Autodesk Inventor part; units mm, degrees
ref_plane "YZ Plane" through (0, 0, 0) normal (1, 0, 0) x (0, 1, 0)
ref_plane "XZ Plane" through (0, 0, 0) normal (0, 1, 0) x (-1, 0, 0)
ref_plane "XY Plane" through (0, 0, 0) normal (0, 0, 1) x (1, 0, 0)
sketch "Sketch1" plane through (0, 0, 0) normal (1, 0, 0) x (0, 1, 0)
  arc A0 (3.7081, 1.5) -> (3.7081, -1.5) centre (0, 0) ccw
  arc A1 (6.5427, 1.6009) -> (8.0964, 0.4688) centre (7.99, 1.955) ccw
  arc A2 (8.0964, -0.4688) -> (6.5427, -1.6009) centre (7.99, -1.955) ccw
  arc A3 (8.0964, -0.4688) -> (8.0964, 0.4688) centre (8.13, 0) ccw
  arc A4 (5.0493, 4.458) -> (6.9512, 4.1777) centre (6.1663, 5.4442) ccw
  arc A5 (7.3869, 3.3475) -> (6.9512, 4.1777) centre (7.1988, 3.7782) ccw
  arc A6 (7.3869, 3.3475) -> (6.5372, 1.623) centre (7.9833, 1.9821) ccw
  arc A7 (2.3992, 6.2939) -> (4.2135, 6.9295) centre (2.9299, 7.6862) ccw
  arc A8 (4.9851, 6.3969) -> (4.2135, 6.9295) centre (4.6184, 6.6909) ccw
  arc A9 (4.9851, 6.3969) -> (5.0342, 4.4751) centre (6.1478, 5.4651) ccw
  arc A10 (-0.8006, 6.688) -> (0.5105, 8.0939) centre (-0.9777, 8.1674) ccw
  arc A11 (1.4413, 7.9809) -> (0.5105, 8.0939) centre (0.98, 8.0707) ccw
  arc A12 (1.4413, 7.9809) -> (2.3778, 6.302) centre (2.9038, 7.6961) ccw
  arc A13 (-3.8169, 5.5498) -> (-3.3094, 7.4041) centre (-4.6612, 6.7775) ccw
  arc A14 (-2.4327, 7.7365) -> (-3.3094, 7.4041) centre (-2.8829, 7.6017) ccw
  arc A15 (-2.4327, 7.7365) -> (-0.8232, 6.6852) centre (-1.0053, 8.164) ccw
  arc A16 (-5.9589, 3.1403) -> (-6.3711, 5.018) centre (-7.277, 3.835) ccw
  arc A17 (-5.7494, 5.7198) -> (-6.3711, 5.018) centre (-6.0854, 5.3912) ccw
  arc A18 (-5.7494, 5.7198) -> (-3.8357, 5.5369) centre (-4.6842, 6.7617) ccw
  arc A19 (-6.7357, 0.0114) -> (-7.9734, 1.4824) centre (-8.2257, 0.0139) ccw
  arc A20 (-7.749, 2.3928) -> (-7.9734, 1.4824) centre (-7.8938, 1.9456) ccw
  arc A21 (-7.749, 2.3928) -> (-5.9695, 3.1201) centre (-7.29, 3.8103) ccw
  arc A22 (-5.9695, -3.1201) -> (-7.749, -2.3928) centre (-7.29, -3.8103) ccw
  arc A23 (-7.9734, -1.4824) -> (-7.749, -2.3928) centre (-7.8938, -1.9456) ccw
  arc A24 (-7.9734, -1.4824) -> (-6.7357, -0.0114) centre (-8.2257, -0.0139) ccw
  arc A25 (-3.8357, -5.5369) -> (-5.7494, -5.7198) centre (-4.6842, -6.7617) ccw
  arc A26 (-6.3711, -5.018) -> (-5.7494, -5.7198) centre (-6.0854, -5.3912) ccw
  arc A27 (-6.3711, -5.018) -> (-5.9589, -3.1403) centre (-7.277, -3.835) ccw
  arc A28 (-0.8232, -6.6852) -> (-2.4327, -7.7365) centre (-1.0053, -8.164) ccw
  arc A29 (-3.3094, -7.4041) -> (-2.4327, -7.7365) centre (-2.8829, -7.6017) ccw
  arc A30 (-3.3094, -7.4041) -> (-3.8169, -5.5498) centre (-4.6612, -6.7775) ccw
  arc A31 (2.3778, -6.302) -> (1.4413, -7.9809) centre (2.9038, -7.6961) ccw
  arc A32 (0.5105, -8.0939) -> (1.4413, -7.9809) centre (0.98, -8.0707) ccw
  arc A33 (0.5105, -8.0939) -> (-0.8006, -6.688) centre (-0.9777, -8.1674) ccw
  arc A34 (5.0342, -4.4751) -> (4.9851, -6.3969) centre (6.1478, -5.4651) ccw
  arc A35 (4.2135, -6.9295) -> (4.9851, -6.3969) centre (4.6184, -6.6909) ccw
  arc A36 (4.2135, -6.9295) -> (2.3992, -6.2939) centre (2.9299, -7.6862) ccw
  arc A37 (6.5372, -1.623) -> (7.3869, -3.3475) centre (7.9833, -1.9821) ccw
  arc A38 (6.9512, -4.1777) -> (7.3869, -3.3475) centre (7.1988, -3.7782) ccw
  arc A39 (6.9512, -4.1777) -> (5.0493, -4.458) centre (6.1663, -5.4442) ccw
  arc A40 (6.5427, 1.6009) -> (6.5372, 1.623) centre (0, 0) ccw
  arc A41 (6.5372, -1.623) -> (6.5427, -1.6009) centre (0, 0) ccw
  arc A42 (5.0493, 4.458) -> (5.0342, 4.4751) centre (0, 0) ccw
  arc A43 (2.3992, 6.2939) -> (2.3778, 6.302) centre (0, 0) ccw
  arc A44 (-0.8006, 6.688) -> (-0.8232, 6.6852) centre (0, 0) ccw
  arc A45 (-3.8169, 5.5498) -> (-3.8357, 5.5369) centre (0, 0) ccw
  arc A46 (-5.9589, 3.1403) -> (-5.9695, 3.1201) centre (0, 0) ccw
  arc A47 (-6.7357, 0.0114) -> (-6.7357, -0.0114) centre (0, 0) ccw
  arc A48 (-5.9695, -3.1201) -> (-5.9589, -3.1403) centre (0, 0) ccw
  arc A49 (-3.8357, -5.5369) -> (-3.8169, -5.5498) centre (0, 0) ccw
  arc A50 (-0.8232, -6.6852) -> (-0.8006, -6.688) centre (0, 0) ccw
  arc A51 (2.3778, -6.302) -> (2.3992, -6.2939) centre (0, 0) ccw
  arc A52 (5.0342, -4.4751) -> (5.0493, -4.458) centre (0, 0) ccw
  line L0 (5.5, 0) -> (5.5, 1.5)
  line L1 (5.5, 1.5) -> (3.7081, 1.5)
  line L2 (3.7081, -1.5) -> (5.5, -1.5)
  line L3 (5.5, -1.5) -> (5.5, 0)
  dimension "d13" = 360
extrude "Extrusion2" add sketch "Sketch1" along normal blind 16
properties part number "MotorGear"
Design review of the part built by this model. Coordinates are the model's own, in mm. A direction names the side the tool comes from. Round coordinates to 2 decimals unless told otherwise and drop trailing zeros. Write each loop counter-clockwise with the first axis right and the second up, starting at its lowest first coordinate (ties: lowest second). Pieces come first, ordered by that corner, then holes. Notation, with made-up numbers: (3.25, 89) - (14.25, 89) arc R17 cw to (14.25, 93) - close; hole circle Ø4 at (-7, -38.75). An arc over 180 degrees is marked (long way). Return JSON: item names as keys, results as strings. Group by question number.
Item 1: The part is to be moulded in two halves that separate along Z. For faces 1 (the face through (7.888, 3.436, 6.285)), 2 (the face through (7.888, -6.444, 5.695)), 3 (the face through (7.9, 8.6, 0)), say which applies: pulls with the +Z half, pulls with the -Z half, needs draft (parallel to the pull), parting line crosses it, or undercut.
Item 2: For probe 1 along Z at (x, y) = (12.5, -6); probe 2 along Z at (x, y) = (14.5, 4); probe 3 along Z at (x, y) = (12, 0), list the stretches that pass through material, from the lowest coordinate up. Write a range as [from, to].
Item 3: We need section B-B on z = -1.25. Write out the cut boundary in (x, y), and give its area (3 significant figures).
Item 4: Machinability: for faces 4 (the face through (7.89, -3.22, 6.4)), 5 (the face through (7.888, -7.095, 0.984)), 6 (the face through (7.888, 4.658, -5.442)), which of the approach directions +Z, -Z, +X, -X, +Y, -Y give a long, thin tool a straight path to every point of the face, cutting with its end or side? Answer none if there is none.
Item 5: Insertion check: P1, Ø0.9, axis at x = 10, y = 4.5, coming from the -Z side; P2, Ø2, axis at x = 2.5, z = -3.5, coming from the -Y side. Each pin has a flat end and moves straight along its axis. Give the tip position at first contact, or say it passes through.
Item 6: We need section A-A on y = 1. Write out the cut boundary in (x, z), and give its area (3 significant figures).
Model answer:
{
 "1": {"face 1": "pulls with the +Z half", "face 2": "undercut", "face 3": "parting line crosses it"},
 "2": {"probe 1": "z = [-5.85, -4.6], [-3.06, 3.06], [4.6, 5.85]", "probe 2": "z = [-6.65, -1.5], [1.5, 6.65]", "probe 3": "z = [-7.04, -4], [4, 7.04]"},
 "3": {"outline": "(0, -7.39) - (16, -7.39) - (16, -3.8) - (0, -3.8) - close; (0, 5.5) - (16, 5.5) - (16, 6.68) - (0, 6.68) - close", "area": "76.3 mm²"},
 "4": {"face 4": "+X, -X", "face 5": "+X, -X, -Y", "face 6": "+X, -X, +Y"},
 "5": {"P1": "stops at z = -7.16", "P2": "stops at y = -6.58"},
 "6": {"outline": "(0, -8.54) - (16, -8.54) - (16, -3.87) - (0, -3.87) - close; (0, 3.87) - (16, 3.87) - (16, 8.54) - (0, 8.54) - close", "area": "149 mm²"}
}
